```python
from build123d import *

# Parameters (mm, degrees)
F0_R     = 2.5
F1_DEPTH = 7
F2_DEPTH = 6
F3_DEPTH = 5


with BuildPart() as f1:
    # F0 (on Front) → F1 (new body)
    with BuildSketch(Plane.XZ):
        Polygon((-22, -76), (0, -76), (22, -76), (22, -70.6540869306), (22, -63), (5, -63), (5, -61.2964109879), (5, -11.9999500107), (5, 0), (5, 40), (5, 63), (8.2548681714, 63), (22, 63), (22, 70.6540869306), (22, 76), (0, 76), (-22, 76), (-22, 70.6540869306), (-22, 63), (-8.2548681714, 63), (-5, 63), (-5, 40), (-5, 0), (-5, -11.9999500107), (-5, -61.2964109879), (-5, -63), (-22, -63), (-22, -70.6540869306), align=None)
        with Locations((0, 69.456204772)):
            Circle(F0_R, mode=Mode.SUBTRACT)
    extrude(amount=F1_DEPTH)

    # F0 (on Front) → F2 (join)
    with BuildSketch(Plane.XZ):
        Polygon((34.9798961949, -50.5831677754), (54.0124350294, -50.5831677754), (63.4277144759, -50.5831677754), (63.4277144759, -38.5831677754), (63.1453811804, -38.5831677754), (51.4277144759, -38.5831677754), (50.1556774178, -35.5901394035), (34.9998075814, 0.0707307999), (9.185549765, 60.8101609562), (8.2548681714, 63), (5, 63), (5, 40), (22, 0), (5, 0), (5, -11.9999500107), (27.307384864, -11.9999500107), (39.0647144759, -38.5831677754), (18.4277144759, -38.5831677754), (18.4277144759, -50.5831677754), align=None)
        Polygon((-63.4277144759, -50.5831677754), (-54.0124350294, -50.5831677754), (-34.9798961949, -50.5831677754), (-18.4277144759, -50.5831677754), (-18.4277144759, -38.5831677754), (-39.0647144759, -38.5831677754), (-27.307384864, -11.9999500107), (-5, -11.9999500107), (-5, 0), (-22, 0), (-5, 40), (-5, 63), (-8.2548681714, 63), (-9.185549765, 60.8101609562), (-34.9998075814, 0.0707307999), (-50.1556774178, -35.5901394035), (-51.4277144759, -38.5831677754), (-63.1453811804, -38.5831677754), (-63.4277144759, -38.5831677754), align=None)
    extrude(amount=F2_DEPTH)

    # F0 (on Front) → F3 (join)
    with BuildSketch(Plane.XZ):
        with BuildLine():
            Line((22, 63), (8.2548681714, 63))
            Line((8.2548681714, 63), (9.185549765, 60.8101609562))
            ThreePointArc((9.185549765, 60.8101609562), (34.068237255, 51.2016133568), (52.542409199, 31.9616212912))
            Line((52.542409199, 31.9616212912), (63.2217606622, 38.4578857813))
            ThreePointArc((63.2217606622, 38.4578857813), (45.5503673388, 58.3194996146), (22, 70.6540869306))
            Line((22, 70.6540869306), (22, 63))
        make_face()
        with BuildLine():
            ThreePointArc((-22, 70.6540869306), (-69.2504760851, 26.0839330237), (-63.1453811804, -38.5831677754))
            Line((-63.1453811804, -38.5831677754), (-51.4277144759, -38.5831677754))
            Line((-51.4277144759, -38.5831677754), (-50.1556774178, -35.5901394035))
            ThreePointArc((-50.1556774178, -35.5901394035), (-56.6003514852, 24.0551493812), (-9.185549765, 60.8101609562))
            Line((-9.185549765, 60.8101609562), (-8.2548681714, 63))
            Line((-8.2548681714, 63), (-22, 63))
            Line((-22, 63), (-22, 70.6540869306))
        make_face()
        with BuildLine():
            ThreePointArc((-54.0124350294, -50.5831677754), (-39.3088160431, -62.6962278075), (-22, -70.6540869306))
            Line((-22, -70.6540869306), (-22, -63))
            Line((-22, -63), (-5, -63))
            Line((-5, -63), (-5, -61.2964109879))
            ThreePointArc((-5, -61.2964109879), (-20.6952028251, -57.9133713406), (-34.9798961949, -50.5831677754))
            Line((-34.9798961949, -50.5831677754), (-54.0124350294, -50.5831677754))
        make_face()
        with BuildLine():
            Line((22, -63), (22, -70.6540869306))
            ThreePointArc((22, -70.6540869306), (39.3088160431, -62.6962278075), (54.0124350294, -50.5831677754))
            Line((54.0124350294, -50.5831677754), (34.9798961949, -50.5831677754))
            ThreePointArc((34.9798961949, -50.5831677754), (20.6952028251, -57.9133713406), (5, -61.2964109879))
            Line((5, -61.2964109879), (5, -63))
            Line((5, -63), (22, -63))
        make_face()
        with BuildLine():
            Line((51.4277144759, -38.5831677754), (63.1453811804, -38.5831677754))
            ThreePointArc((63.1453811804, -38.5831677754), (63.1836019728, -38.5205457093), (63.2217606622, -38.4578857813))
            Line((63.2217606622, -38.4578857813), (52.542409199, -31.9616212912))
            ThreePointArc((52.542409199, -31.9616212912), (51.3810839182, -33.7969557118), (50.1556774178, -35.5901394035))
            Line((50.1556774178, -35.5901394035), (51.4277144759, -38.5831677754))
        make_face()
    extrude(amount=F3_DEPTH)


solid = f1.part
```
Geometry: final body of the model. Coordinates: model frame, mm. A direction names the side the tool comes from. Coordinates: 2 decimals unless noted, no trailing zeros. Loops run counter-clockwise (first coordinate to the right, second up) from the corner with the lowest first, then second, coordinate; pieces in that order, holes last. Notation, with made-up numbers: M 12.5,6 L 61.5,6 A31 cw 61.5,37 Z; hole C 15.5,-22.5 d11. An arc over 180 degrees is marked long. Put each result on its own line as item: value.
(1) Draft query along X for faces 5 (the face through (45.84, -2.46, 58.09)), 6 (the face through (-30, -5, -58)), 7 (the face through (-22, -4, 71)), 8 (the face through (18.428, -3, -44)). Return one class per face: pulls with the +X half, pulls with the -X half, needs draft (parallel to the pull), parting line crosses it, or undercut.
Answer sheet:
face 5: pulls with the +X half
face 6: needs draft
face 7: pulls with the -X half
face 8: undercut
(2) Cut plane A-A on x = 0. Return the cut outline in (y, z), then the cut area to 3 significant figures.
Answer sheet:
outline: M -7,-76 L 0,-76 L 0,66.96 L -7,66.96 Z; M -7,71.96 L 0,71.96 L 0,76 L -7,76 Z
area: 1,030 mm^2
(3) Material intervals for probe 1 along X at (y, z) = (-4.75, -44); probe 2 along Z at (x, y) = (0, -3.5); probe 3 along X at (y, z) = (-1, -53), sorted ascending.
Answer sheet:
probe 1: x = -63.43 to -18.43, -5 to 5, 18.43 to 63.43
probe 2: z = -76 to 66.96, 71.96 to 76
probe 3: x = -51.64 to -31.2, -5 to 5, 31.2 to 51.64
(4) First-contact query: pin 1 (3 mm diameter, centred on x = 37.5, y = -3.5, fed in from -Z); pin 2 (2 mm diameter, centred on y = -5, z = 69, fed in from -X); pin 3 (3 mm diameter, centred on x = 41.5, y = -1.5, fed in from +Z). Flat tips, straight axial feed; report the tip coordinate or a pass-through.
Answer sheet:
pin 1: stops at z = -64.65
pin 2: stops at x = -29.19
pin 3: stops at z = 62.26
(5) Access query for faces 1 (the face through (30, -6, -6)), 2 (the face through (57.807, -2.465, 35.164)), 3 (the face through (-13.62, -2.96, 19.72)), 4 (the face through (22, -4, 71)). Directions: +Z, -Z, +X, -X, +Y, -Y. A direction counts if a zero-diameter tool reaches every point of the face in a straight line with its end or side. Return the directions, or none.
Answer sheet:
face 1: +X, -Y
face 2: +X, +Y, -Y
face 3: +Y, -Y
face 4: +Z, +X, -Y
(6) Cut plane B-B on z = 56. Return the cut outline in (x, y).
Answer sheet:
outline: M -48.37,-5 L -25.42,-5 L -25.42,0 L -48.37,0 Z; M -11.23,-6 L -5,-6 L -5,-7 L 5,-7 L 5,-6 L 11.23,-6 L 11.23,0 L -11.23,0 Z; M 25.42,-5 L 48.37,-5 L 48.37,0 L 25.42,0 Z
(7) Cut plane D-D on x = -56.5. Return the cut outline in (y, z), then the cut area to 3 significant figures.
Answer sheet:
outline: M -6,-50.58 L 0,-50.58 L 0,-24.29 L -5,-24.29 L -5,-38.58 L -6,-38.58 Z; M -5,24.29 L 0,24.29 L 0,47.79 L -5,47.79 Z
area: 261 mm^2
(8) Cut plane C-C on x = -32.5. Return the cut outline in (y, z), then the cut area to 3 significant figures.
Answer sheet:
outline: M -6,-50.58 L 0,-50.58 L 0,-38.58 L -6,-38.58 Z; M -6,-23.74 L 0,-23.74 L 0,5.95 L -6,5.95 Z; M -5,-66.48 L 0,-66.48 L 0,-52.21 L -5,-52.21 Z; M -5,52.21 L 0,52.21 L 0,66.48 L -5,66.48 Z
area: 393 mm^2
